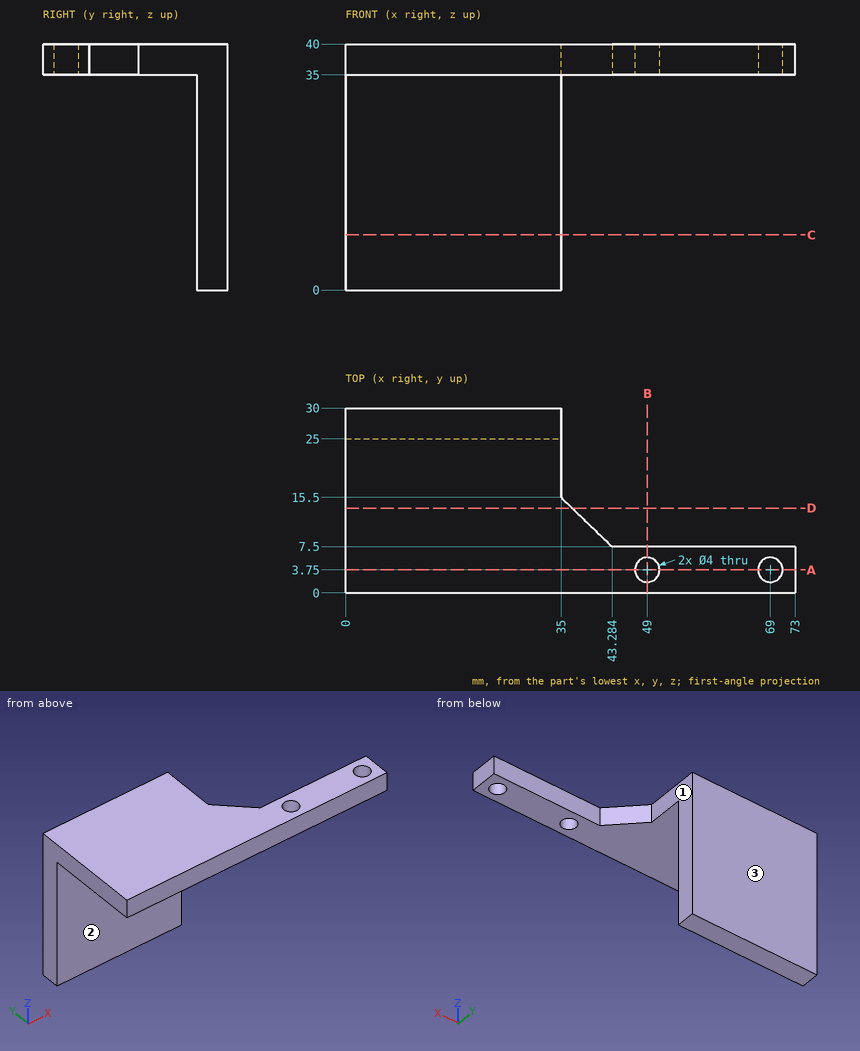
Drawing for the job (mm, zero at the part's lowest x, y, z). A direction names the side the tool comes from. Round coordinates to 2 decimals unless told otherwise and drop trailing zeros. Order: outer loops, then holes, each group sorted by start corner. A loop starts at its lowest first (then second) coordinate and runs counter-clockwise, first axis right, second up. Notation, with made-up numbers: M 15,10.25 L 74,10.25 A18 ccw 74,18.25 Z; hole C 70,26.5 d5. An arc over 180 degrees is marked long. Use one line per item in the form item = value.
Q1. Saw through at A-A on y = 3.75. Give the cut face in (x, z), then the cut area to 3 significant figures.
Recorded:
outline = M 0,35 L 47,35 L 47,40 L 0,40 Z; M 51,35 L 67,35 L 67,40 L 51,40 Z; M 71,35 L 73,35 L 73,40 L 71,40 Z
area = 325 mm^2
Q2. Saw through at D-D on y = 13.75. Give the cut face in (x, z).
Recorded:
outline = M 0,35 L 36.81,35 L 36.81,40 L 0,40 Z
Q3. Which spindle directions (+Z, -Z, +X, -X, +Y, -Y) get a long thin tool onto all of the face, cutting with end or side? Do the marked faces 1, 2 and 3. Say none if no direction does.
Recorded:
face_1 = +Z, -Z, +X, +Y
face_2 = -Z, +X, -X, -Y
face_3 = +Z, -Z, +X, -X, +Y
Q4. Saw through at B-B on x = 49. Give the cut face in (y, z), then the cut area to 3 significant figures.
Recorded:
outline = M 0,35 L 1.75,35 L 1.75,40 L 0,40 Z; M 5.75,35 L 7.5,35 L 7.5,40 L 5.75,40 Z
area = 17.5 mm^2
Q5. Saw through at C-C on z = 9. Give the cut face in (x, y).
Recorded:
outline = M 0,25 L 35,25 L 35,30 L 0,30 Z
Q6. Probe L1, parallel to Y at x = 49, z = 37; L2, parallel to X at y = 27.5, z = 14; L3, parallel to Y at x = 12.5, z = 7. List the from-to ranges inside material, lowest first.
Recorded:
L1 = 0 to 1.75, 5.75 to 7.5
L2 = 0 to 35
L3 = 25 to 30
Q7. Flat gauge pins, fed straight in: P1, Ø2.5, axis at x = 65, z = 36.5, coming from the +Y side; P2, Ø10.5, axis at x = 18, z = 19, coming from the -Y side; P3, Ø3, axis at x = 31.5, y = 20, coming from the -Z side; P4, Ø4.5, axis at y = 21, z = 25, coming from the +X side. Where does each tip first touch, or does it go through?
Recorded:
P1 = 7.5
P2 = 25
P3 = 35
P4 = through
